Can you work these out from the model? Positions are in its coordinate system, mm. A direction names the side the tool comes from. Round coordinates to 2 decimals unless told otherwise and drop trailing zeros. Order: outer loops, then holes, each group sorted by start corner. A loop starts at its lowest first (then second) coordinate and runs counter-clockwise, first axis right, second up. Notation, with made-up numbers: M 9,14 L 45,14 A24 ccw 45,45 Z; hole C 56.5,-23.75 d9. An arc over 180 degrees is marked long. Answer as a JSON object with one key per item and string values. Group by question number.
Autodesk Inventor part; units mm, degrees
ref_plane "YZ Plane" through (0, 0, 0) normal (1, 0, 0) x (0, 1, 0)
ref_plane "XZ Plane" through (0, 0, 0) normal (0, 1, 0) x (-1, 0, 0)
ref_plane "XY Plane" through (0, 0, 0) normal (0, 0, 1) x (1, 0, 0)
sketch "Sketch1" plane through (0, 0, 0) normal (0, 1, 0) x (-1, 0, 0)
  line L0 (34.6075, 19.4945) -> (-34.6075, 19.4945)
  line L1 (-34.6075, 19.4945) -> (-34.6075, -19.4945)
  line L2 (-34.6075, -19.4945) -> (34.6075, -19.4945)
  line L3 (34.6075, -19.4945) -> (34.6075, 19.4945)
  line L4 (-34.6075, 19.4945) -> (34.6075, -19.4945) construction
  circle A0 centre (32.4355, 0.7215) radius 1.75
  circle A1 centre (-32.4485, 0.7215) radius 1.75
  line L5 (28.7695, 5.2375) -> (1.7695, 5.2375)
  line L6 (1.7695, 5.2375) -> (1.7695, -4.7625)
  line L7 (1.7695, -4.7625) -> (28.7695, -4.7625)
  line L8 (28.7695, -4.7625) -> (28.7695, 5.2375)
  line L9 (28.7695, 5.2375) -> (1.7695, -4.7625) construction
  line L10 (1.7695, 5.2375) -> (28.7695, -4.7625) construction
  line L11 (-28.7695, 5.2375) -> (-1.7695, 5.2375)
  line L12 (-1.7695, 5.2375) -> (-1.7695, -4.7625)
  line L13 (-1.7695, -4.7625) -> (-28.7695, -4.7625)
  line L14 (-28.7695, -4.7625) -> (-28.7695, 5.2375)
  point P0 (0, 0)
  point P1 (15.2695, 0.2375)
  dimension "d0" = 69.215
  dimension "d1" = 38.989
  dimension "d2" = 3.5
  dimension "d3" = 2.172
  dimension "d4" = 20.216
  dimension "d5" = 27
  dimension "d6" = 10
  dimension "d18" = 64.884
extrude "Extrusion1" add sketch "Sketch1" along normal blind 1.7
extrude "Extrusion2" add sketch "Sketch1" along normal blind 16.58 contours L8 L7 L6 L5 | L11 L12 L13 L14
sketch "Sketch2" plane through (0, 1.7, 0) normal (0, 1, 0) x (1, 0, 0)
  line L0 (-16.1466, -9.4421) -> (18.9981, -9.4421) construction
  line L1 (18.9981, -9.4421) -> (18.9981, -13.0896) construction
  line L2 (18.9981, -13.0896) -> (-16.1466, -13.0896) construction
  line L3 (-16.1466, -13.0896) -> (-16.1466, -9.4421) construction
  point P0 (0, 0)
properties part number "powerdistv2"
Item 1: Suppose I cut it at A-A, the plane y = 15.75. Write out the boundary of the cut face in (x, z).
Item 2: If we mould it in two halves opening along X, with no side actions, what happens to faces 6 (the face through (-15, 16.58, 0)), 7 (the face through (34.197, 0.838, 0.645)), 8 (the face through (-28.77, 9, 0))? For each: +X half, -X half, draft (parallel to the pull), parting line (faces both ways), or undercut.
Item 3: Suppose I cut it at C-C, the plane z = -2.5. Write out the boundary of the cut face in (x, y), and give its area (3 significant figures).
Item 4: I need wall thicknesses on line 1 (X direction, y = 6, z = 4); line 2 (Y direction, x = -27, z = -15.5); line 3 (Z direction, x = -7, y = 4.75). Which ranges of each line are inside material? Lowest first, please.
Item 5: I'm going to push flat-ended pins straight in: pin 1 Ø4.5 at (x, y) = (-12.5, 11.5) entering from +Z; pin 2 Ø8 at (y, z) = (13, -2) entering from +X; pin 3 Ø5.5 at (x, z) = (32.45, 0.72) entering from +Y. Where does each tip first touch, or does it pass through?
Item 6: Suppose I cut it at D-D, the plane z = 9. Write out the boundary of the cut face in (x, y), and give its area (3 significant figures).
Item 7: Suppose I cut it at B-B, the plane x = 26. Write out the boundary of the cut face in (y, z).
Item 8: On a 3-axis mill with a long thin cutter (end or side, diameter ignored), from which of +Z, -Z, +X, -X, +Y, -Y can I reach the whole of each face in a straight line? I mean faces 1 (the face through (0, 0, 0)), 2 (the face through (15, 9, 5.238)), 3 (the face through (1.77, 9, 0)), 4 (the face through (28.77, 9, 0)), 5 (the face through (15, 9, -4.762)). Say none if no direction works.
Computed:
{
 "1": {"outline": "M -28.77,-4.76 L -1.77,-4.76 L -1.77,5.24 L -28.77,5.24 Z; M 1.77,-4.76 L 28.77,-4.76 L 28.77,5.24 L 1.77,5.24 Z"},
 "2": {"face 6": "draft", "face 7": "undercut", "face 8": "-X half"},
 "3": {"outline": "M -34.61,0 L 34.61,0 L 34.61,1.7 L 28.77,1.7 L 28.77,16.58 L 1.77,16.58 L 1.77,1.7 L -1.77,1.7 L -1.77,16.58 L -28.77,16.58 L -28.77,1.7 L -34.61,1.7 Z", "area": "921 mm^2"},
 "4": {"line 1": "x = -28.77 to -1.77, 1.77 to 28.77", "line 2": "y = 0 to 1.7", "line 3": "z = -4.76 to 5.24"},
 "5": {"pin 1": "stops at z = 5.24", "pin 2": "stops at x = 28.77", "pin 3": "stops at y = 1.7"},
 "6": {"outline": "M -34.61,0 L 34.61,0 L 34.61,1.7 L -34.61,1.7 Z", "area": "118 mm^2"},
 "7": {"outline": "M 0,-19.49 L 1.7,-19.49 L 1.7,-4.76 L 16.58,-4.76 L 16.58,5.24 L 1.7,5.24 L 1.7,19.49 L 0,19.49 Z"},
 "8": {"face 1": "+Z, -Z, +X, -X, -Y", "face 2": "+Z, +X, -X, +Y", "face 3": "+Z, -Z, +Y", "face 4": "+Z, -Z, +X, +Y", "face 5": "-Z, +X, -X, +Y"}
}
